from build123d import *

# Parameters (mm, degrees)
SKETCH1_W                  = 82
SKETCH1_H                  = 10
SKETCH1_R                  = 2
BASE_FLANGE1_DEPTH         = 4
SKETCHED_START             = -5
SKETCHED_BEND1_DEPTH       = 10
SKETCHED_BEND1_2_DEPTH     = 2.9999999
SKETCHED_START_2           = 2.0000001
SKETCHED_BEND1_3_DEPTH     = 2.9999999
SKETCHED_START_3           = -2.0000001
SKETCHED_BEND1_4_DEPTH     = 4.0000002
SKETCHED_START_4           = -28
SKETCHED_BEND1_5_OUTLINE_R = 2
SKETCHED_BEND1_5_DEPTH     = 56


with BuildPart() as part:
    # Base-Flange1: sheet metal written as solids
    # Sketch1 → Base-Flange1 (new body)
    with BuildSketch(Plane(origin=(0, 0, 0), x_dir=(1, 0, 0), z_dir=(0, 1, 0))):
        Rectangle(SKETCH1_W, SKETCH1_H)
        with Locations(Location((14, 0, 0), (0, 0, 270))):
            Circle(SKETCH1_R, mode=Mode.SUBTRACT)
        with Locations(Location((35, 0, 0), (0, 0, 270))):
            Circle(SKETCH1_R, mode=Mode.SUBTRACT)
        with Locations(Location((-35, 0, 0), (0, 0, 90))):
            Circle(SKETCH1_R, mode=Mode.SUBTRACT)
        with Locations(Location((-14, 0, 0), (0, 0, 90))):
            Circle(SKETCH1_R, mode=Mode.SUBTRACT)
    extrude(amount=-BASE_FLANGE1_DEPTH)

    # Sketched Bend1: read off the stored shape, not the designer's step
    # Sketched Bend1 outline → Sketched Bend1 (cut)
    with BuildSketch(Plane.XY.offset(SKETCHED_START)):
        with BuildLine():
            ThreePointArc((20, 0), (23.999999999, -1.07179677), (26.92820323, -4))
            Line((26.92820323, -4), (41, -4))
            Line((41, -4), (41, 0))
            Line((41, 0), (20, 0))
        make_face()
        with BuildLine():
            Line((-41, -4), (-26.92820323, -4))
            ThreePointArc((-26.92820323, -4), (-23.999999999, -1.07179677), (-20, 0))
            Line((-20, 0), (-41, 0))
            Line((-41, 0), (-41, -4))
        make_face()
    extrude(amount=SKETCHED_BEND1_DEPTH, mode=Mode.SUBTRACT)

    # Sketched Bend1 2 outline → Sketched Bend1 2 (add)
    with BuildSketch(Plane.XY.offset(SKETCHED_START)):
        with BuildLine():
            ThreePointArc((20, -4), (22.828427125, -5.171572875), (24, -8))
            Line((24, -8), (24, -19.575222039))
            Line((24, -19.575222039), (28, -19.575222039))
            Line((28, -19.575222039), (28, -8))
            ThreePointArc((28, -8), (27.72740661, -5.929447639), (26.92820323, -4))
            Line((26.92820323, -4), (20, -4))
        make_face()
        with BuildLine():
            ThreePointArc((-24, -8), (-22.828427125, -5.171572875), (-20, -4))
            Line((-20, -4), (-26.92820323, -4))
            ThreePointArc((-26.92820323, -4), (-27.72740661, -5.929447639), (-28, -8))
            Line((-28, -8), (-28, -19.575222039))
            Line((-28, -19.575222039), (-24, -19.575222039))
            Line((-24, -19.575222039), (-24, -8))
        make_face()
    extrude(amount=SKETCHED_BEND1_2_DEPTH)

    # Sketched Bend1 3 outline → Sketched Bend1 3 (add)
    with BuildSketch(Plane.XY.offset(SKETCHED_START_2)):
        with BuildLine():
            ThreePointArc((20, -4), (22.828427125, -5.171572875), (24, -8))
            Line((24, -8), (24, -19.575222039))
            Line((24, -19.575222039), (28, -19.575222039))
            Line((28, -19.575222039), (28, -8))
            ThreePointArc((28, -8), (27.72740661, -5.929447639), (26.92820323, -4))
            Line((26.92820323, -4), (20, -4))
        make_face()
        with BuildLine():
            ThreePointArc((-24, -8), (-22.828427125, -5.171572875), (-20, -4))
            Line((-20, -4), (-26.92820323, -4))
            ThreePointArc((-26.92820323, -4), (-27.72740661, -5.929447639), (-28, -8))
            Line((-28, -8), (-28, -19.575222039))
            Line((-28, -19.575222039), (-24, -19.575222039))
            Line((-24, -19.575222039), (-24, -8))
        make_face()
    extrude(amount=SKETCHED_BEND1_3_DEPTH)

    # Sketched Bend1 4 outline → Sketched Bend1 4 (add)
    with BuildSketch(Plane.XY.offset(SKETCHED_START_3)):
        with BuildLine():
            ThreePointArc((-24, -8), (-22.828427125, -5.171572875), (-20, -4))
            Line((-20, -4), (-26.92820323, -4))
            ThreePointArc((-26.92820323, -4), (-27.72740661, -5.929447639), (-28, -8))
            Line((-28, -8), (-28, -19.575222039))
            Line((-28, -19.575222039), (-24, -19.575222039))
            Line((-24, -19.575222039), (-24, -8))
        make_face()
        with BuildLine():
            ThreePointArc((20, -4), (22.828427125, -5.171572875), (24, -8))
            Line((24, -8), (24, -19.575222039))
            Line((24, -19.575222039), (28, -19.575222039))
            Line((28, -19.575222039), (28, -8))
            ThreePointArc((28, -8), (27.72740661, -5.929447639), (26.92820323, -4))
            Line((26.92820323, -4), (20, -4))
        make_face()
    extrude(amount=SKETCHED_BEND1_4_DEPTH)

    # Sketched Bend1 5 outline → Sketched Bend1 5 (cut)
    with BuildSketch(Plane.YZ.offset(SKETCHED_START_4)):
        with Locations((-13.575222039, 0)):
            Circle(SKETCHED_BEND1_5_OUTLINE_R)
    extrude(amount=SKETCHED_BEND1_5_DEPTH, mode=Mode.SUBTRACT)


solid = part.part
Geometry check sheet. Reference: the model listing, model coordinates, mm. A direction names the side the tool comes from. Give positions to 0.01 mm unless a question says otherwise; leave off trailing zeros. Write each loop counter-clockwise with the first axis right and the second up, starting at its lowest first coordinate (ties: lowest second). Pieces come first, ordered by that corner, then holes. Notation, with made-up numbers: (53, -4.5) - (86, -4.5) arc R17 cw to (86, 2.5) - close; hole circle Ø11 at (-19, 46.25). An arc over 180 degrees is marked (long way). Put each result on its own line as item: value.
1. Sectioned sample at A-A, the plane z = 0. Enter the section's corners in (x, y).
Ans:
outline: (-28, -19.58) - (-24, -19.58) - (-24, -15.58) - (-28, -15.58) - close; (-28, -11.58) - (-24, -11.58) - (-24, -8) arc R4 cw to (-20, -4) - (-16, -4) - (-16, 0) - (-20, 0) arc R8 ccw to (-28, -8) - close; (-12, -4) - (12, -4) - (12, 0) - (-12, 0) - close; (16, -4) - (20, -4) arc R4 cw to (24, -8) - (24, -11.58) - (28, -11.58) - (28, -8) arc R8 ccw to (20, 0) - (16, 0) - close; (24, -19.58) - (28, -19.58) - (28, -15.58) - (24, -15.58) - close
2. Draft check along Y on faces 3 (the cylindrical face through (25.972, -15.573, 0.088)), 4 (the flat face through (-26, -19.575, 0)), 5 (the flat face through (0, -3, -5)). Enter one of: +Y half, -Y half, draft (parallel to the pull), parting line (faces both ways), or undercut.
Ans:
face 3: undercut
face 4: -Y half
face 5: draft
3. Thickness scan on line 1 (X direction, y = -16, z = 1); line 2 (X direction, y = -2.75, z = 1.25); line 3 (Z direction, x = -14, y = -1.55). Record the ranges inside material, lowest first.
Ans:
line 1: x = -28 to -24, 24 to 28
line 2: x = -26.04 to -15.56, -12.44 to 12.44, 15.56 to 26.04
line 3: z = -5 to -2, 2 to 5
4. Set-up check for faces 1 (the flat face through (24, -13.7, -2.3)), 2 (the flat face through (0, 0, 0)): record each of +Z, -Z, +X, -X, +Y, -Y from which the full face is reachable in a straight line by a thin tool's end or side.
Ans:
face 1: +Z, -Z, -Y
face 2: +Z, -Z, +X, -X, +Y
5. Go/stop test with flat-tipped pins: pin 1 (2 mm diameter, centred on y = -2.5, z = -1.5, fed in from -X); pin 2 (2.5 mm diameter, centred on x = 14, z = 0, fed in from +Y); pin 3 (4.5 mm diameter, centred on y = -13.58, z = 0, fed in from -X); pin 4 (3 mm diameter, centred on x = 5, z = -1, fed in from -Y). Record where each tip stops, or that it passes through.
Ans:
pin 1: stops at x = -26.61
pin 2: passes through
pin 3: stops at x = -28
pin 4: stops at y = -4
6. Sectioned sample at D-D, the plane z = 2.75. Enter the section's corners in (x, y).
Ans:
outline: (-28, -19.58) - (-24, -19.58) - (-24, -8) arc R4 cw to (-20, -4) - (20, -4) arc R4 cw to (24, -8) - (24, -19.58) - (28, -19.58) - (28, -8) arc R8 ccw to (20, 0) - (-20, 0) arc R8 ccw to (-28, -8) - close
7. Sectioned sample at C-C, the plane x = 14. Enter the section's corners in (y, z).
Ans:
outline: (-4, -5) - (0, -5) - (0, -2) - (-4, -2) - close; (-4, 2) - (0, 2) - (0, 5) - (-4, 5) - close
8. Sectioned sample at B-B, the plane y = -10.25. Enter the section's corners in (x, z), plus the area to 3 significant figures.
Ans:
outline: (-28, -5) - (-24, -5) - (-24, 5) - (-28, 5) - close; (24, -5) - (28, -5) - (28, 5) - (24, 5) - close
area: 80.0 mm²
